Geometry check sheet. Reference: the model listing, model coordinates, mm. Face numbers are marked on the shaded views. A direction names the side the tool comes from. Coordinates: 2 decimals unless noted, no trailing zeros. Write each loop counter-clockwise with the first axis right and the second up, starting at its lowest first coordinate (ties: lowest second). Pieces come first, ordered by that corner, then holes. Notation, with made-up numbers: M 47.25,64.5 L 99.25,64.5 A21 cw 99.25,73.5 Z; hole C 4.5,29.5 d8. An arc over 180 degrees is marked long. Answer as a JSON object with one key per item and string values. Group by question number.
```python
from build123d import *

# Parameters (mm, degrees)
F1_DEPTH  = 280
F2_SIZE   = 5
F3_W      = 931
F3_H      = 526
F4_DEPTH  = 2
F5_R      = 1.5
F6_DEPTH  = 10
F7_W      = 15
F7_H      = 250
F7_W_2    = 125
F8_DEPTH  = 20
F9_W      = 28
F9_H      = 28
F10_DEPTH = 5


with BuildPart() as f1:
    # F0 (on Top) → F1 (new body, symmetric)
    with BuildSketch(Plane.XY):
        with BuildLine():
            Line((-480, -23.964466), (-476.464466, -27.5))
            Line((-476.464466, -27.5), (0, -27.5))
            Line((0, -27.5), (0, 27.5))
            Line((0, 27.5), (-325, 27.5))
            ThreePointArc((-325, 27.5), (-350.22325, 25.818315), (-375, 20.803028))
            ThreePointArc((-375, 20.803028), (-392.520175, 10.560332), (-412.5, 7))
            Line((-412.5, 7), (-430, 7))
            ThreePointArc((-430, 7), (-457.11747, 1.534044), (-480, -14.010205))
            Line((-480, -14.010205), (-480, -23.964466))
        make_face()
        with BuildLine():
            Line((0, 27.5), (0, -27.5))
            Line((0, -27.5), (476.464466, -27.5))
            Line((476.464466, -27.5), (480, -23.964466))
            Line((480, -23.964466), (480, -14.010205))
            ThreePointArc((480, -14.010205), (457.11747, 1.534044), (430, 7))
            Line((430, 7), (412.5, 7))
            ThreePointArc((412.5, 7), (392.520175, 10.560332), (375, 20.803028))
            ThreePointArc((375, 20.803028), (350.22325, 25.818315), (325, 27.5))
            Line((325, 27.5), (0, 27.5))
        make_face()
    extrude(amount=F1_DEPTH, both=True)

    # F2
    f2_edges = [f1.edges().sort_by_distance(p)[0] for p in [
        (0, -27.5, 280),
        (0, -27.5, -280),
    ]]
    chamfer(f2_edges, length=F2_SIZE)

    # F3 (on face) → F4 (cut)
    with BuildSketch(Plane.XZ.offset(27.5)):
        with Locations((0, 2.5)):
            Rectangle(F3_W, F3_H)
    extrude(amount=-F4_DEPTH, mode=Mode.SUBTRACT)

    # F5 (on face) → F6 (cut)
    with BuildSketch(Plane(origin=(0, 27.5, 0), x_dir=(-1, 0, 0), z_dir=(0, 1, 0))):
        with Locations((-200, 228)):
            Circle(F5_R)
        with Locations((200, 228)):
            Circle(F5_R)
        with Locations((200, -172)):
            Circle(F5_R)
        with Locations((-200, -172)):
            Circle(F5_R)
    extrude(amount=-F6_DEPTH, mode=Mode.SUBTRACT)

    # F7 (on face) → F8 (cut)
    with BuildSketch(Plane(origin=(0, 27.5, 0), x_dir=(-1, 0, 0), z_dir=(0, 1, 0))):
        with Locations((332.5, 20)):
            Rectangle(F7_W, F7_H)
        with Locations((262.5, 20)):
            Rectangle(F7_W_2, F7_H)
    extrude(amount=-F8_DEPTH, mode=Mode.SUBTRACT)

    # F9 (on face) → F10 (cut)
    with BuildSketch(Plane(origin=(0, 27.5, 0), x_dir=(-1, 0, 0), z_dir=(0, 1, 0))):
        with Locations((-146, -56)):
            Rectangle(F9_W, F9_H)
    extrude(amount=-F10_DEPTH, mode=Mode.SUBTRACT)


solid = f1.part
```
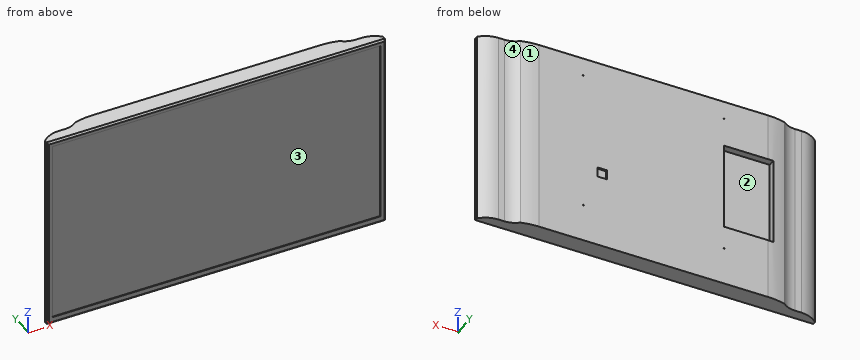
1) Section check A-A (x = 291.5). Record the cut outline in (y, z), then the cut area to 3 significant figures.
2) Draft check along Z on the marked faces 3 and 4. Enter one of: +Z half, -Z half, draft (parallel to the pull), parting line (faces both ways), or undercut.
3) Section check B-B (z = -245.5). Record the cut outline in (x, y).
4) Material ranges on probe 1 along Z at (x, y) = (200, 21.5); probe 2 along Y at (x, z) = (172, 177); probe 3 along X at (y, z) = (20, 228), recorded low to high. Write a range as [from, to].
5) Section check C-C (x = -225). Record the cut outline in (y, z), then the cut area to 3 significant figures.
6) Set-up check for the marked faces 1 and 2: record each of +Z, -Z, +X, -X, +Y, -Y from which the full face is reachable in a straight line by a thin tool's end or side.
7) Go/stop test with flat-tipped pins: pin 1 Ø2 at (y, z) = (1, 15.5) entering from -X; pin 2 Ø1 at (x, z) = (-139, 198.5) entering from -Y; pin 3 Ø1.6 at (y, z) = (-26.5, -76) entering from +X. Record where each tip stops, or that it passes through.
8) Section check D-D (z = -32). Record the cut outline in (x, y), then the cut area to 3 significant figures.
Entries:
{
 "1": {"outline": "M -27.5,-275 L -22.5,-280 L 27.5,-280 L 27.5,280 L -22.5,280 L -27.5,275 L -27.5,265.5 L -25.5,265.5 L -25.5,-260.5 L -27.5,-260.5 Z", "area": "29,700 mm^2"},
 "2": {"face 3": "undercut", "face 4": "draft"},
 "3": {"outline": "M -480,-23.96 L -476.46,-27.5 L -465.5,-27.5 L -465.5,-25.5 L 465.5,-25.5 L 465.5,-27.5 L 476.46,-27.5 L 480,-23.96 L 480,-14.01 A70 ccw 430,7 L 412.5,7 A57.84 cw 375,20.8 A190 ccw 325,27.5 L -325,27.5 A190 ccw -375,20.8 A57.84 cw -412.5,7 L -430,7 A70 ccw -480,-14.01 Z"},
 "4": {"probe 1": "[-280, -173.5], [-170.5, 226.5], [229.5, 280]", "probe 2": "[-25.5, 27.5]", "probe 3": "[-375.96, -201.5], [-198.5, 198.5], [201.5, 375.96]"},
 "5": {"outline": "M -27.5,-275 L -22.5,-280 L 27.5,-280 L 27.5,-105 L 7.5,-105 L 7.5,145 L 27.5,145 L 27.5,280 L -22.5,280 L -27.5,275 L -27.5,265.5 L -25.5,265.5 L -25.5,-260.5 L -27.5,-260.5 Z", "area": "24,700 mm^2"},
 "6": {"face 1": "+Z, -Z, +X, +Y", "face 2": "+Y"},
 "7": {"pin 1": "x = -460.51", "pin 2": "y = -25.5", "pin 3": "x = 478.26"},
 "8": {"outline": "M -480,-23.96 L -476.46,-27.5 L -465.5,-27.5 L -465.5,-25.5 L 465.5,-25.5 L 465.5,-27.5 L 476.46,-27.5 L 480,-23.96 L 480,-14.01 A70 ccw 430,7 L 412.5,7 A57.84 cw 375,20.8 A190 ccw 325,27.5 L -200,27.5 L -200,7.5 L -340,7.5 L -340,26.91 A190 ccw -375,20.8 A57.84 cw -412.5,7 L -430,7 A70 ccw -480,-14.01 Z", "area": "43,300 mm^2"}
}
